For this review, use the dimensioned drawing (mm, ordinates from the lowest corner) and the shaded views. Coordinates: 2 decimals unless noted, no trailing zeros. Loops run counter-clockwise (first coordinate to the right, second up) from the corner with the lowest first, then second, coordinate; pieces in that order, holes last. Notation, with made-up numbers: (-31.75, 45) - (6.25, 45) arc R9 cw to (6.25, 57) - close; hole circle Ø6 at (9, -11). An arc over 180 degrees is marked (long way). One line per item, written item: value. Start each with the question number.
1. We need section B-B, the plane z = 4. Give the boundary of the cut face in (x, y), then the cut area to 3 significant figures.
2. We need section A-A, the plane y = 1.45. Give the boundary of the cut face in (x, z), then the cut area to 3 significant figures.
3. Insertion check: P1, Ø2.5, axis at y = 2, z = 8, coming from the -X side; P2, Ø0.8, axis at x = 145.5, y = 2, coming from the -Z side. Each pin has a flat end and moves straight along its axis. Give the tip position at first contact, or say it passes through.
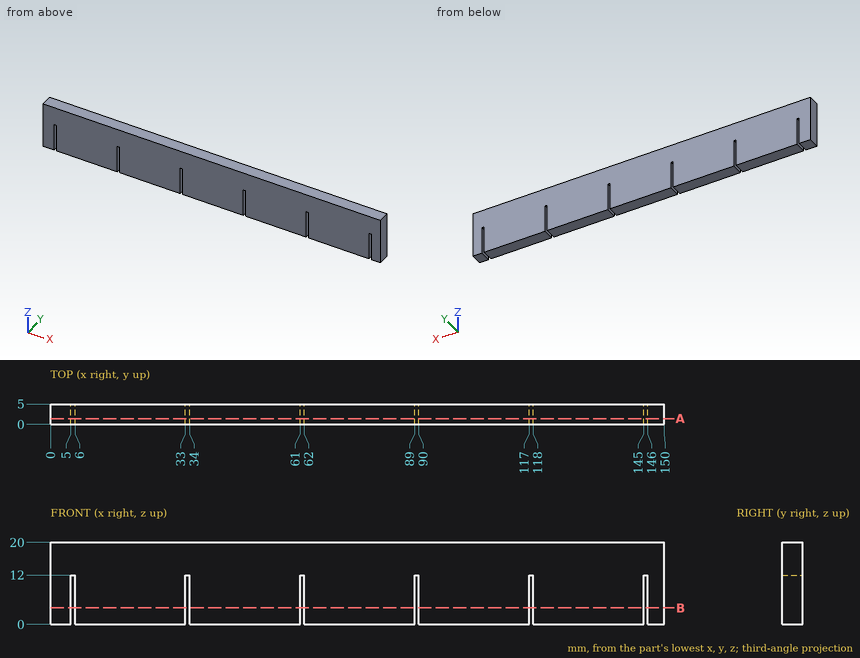
Findings below:
1. outline: (0, 0) - (5, 0) - (5, 5) - (0, 5) - close; (6, 0) - (33, 0) - (33, 5) - (6, 5) - close; (34, 0) - (61, 0) - (61, 5) - (34, 5) - close; (62, 0) - (89, 0) - (89, 5) - (62, 5) - close; (90, 0) - (117, 0) - (117, 5) - (90, 5) - close; (118, 0) - (145, 0) - (145, 5) - (118, 5) - close; (146, 0) - (150, 0) - (150, 5) - (146, 5) - close
1. area: 720 mm2
2. outline: (0, 0) - (5, 0) - (5, 12) - (6, 12) - (6, 0) - (33, 0) - (33, 12) - (34, 12) - (34, 0) - (61, 0) - (61, 12) - (62, 12) - (62, 0) - (89, 0) - (89, 12) - (90, 12) - (90, 0) - (117, 0) - (117, 12) - (118, 12) - (118, 0) - (145, 0) - (145, 12) - (146, 12) - (146, 0) - (150, 0) - (150, 20) - (0, 20) - close
2. area: 2,930 mm2
3. P1: x = 0
3. P2: z = 12
